The model under review builds one solid part; all positions refer to its coordinate system, in mm. A direction names the side the tool comes from. Coordinates: 2 decimals unless noted, no trailing zeros. Order: outer loops, then holes, each group sorted by start corner. A loop starts at its lowest first (then second) coordinate and runs counter-clockwise, first axis right, second up. Notation, with made-up numbers: M 31.5,0.5 L 89.5,0.5 A16 ccw 89.5,21.5 Z; hole C 70,11.25 d6. An arc over 180 degrees is marked long. One line per item, written item: value.
```python
from build123d import *

# Parameters (mm, degrees)
SKETCH1_W                   = 126
SKETCH1_H                   = 5
ENCAIXE_START               = -7
ENCAIXE_POTENCI_METRO_DEPTH = 7


with BuildPart() as part:
    # Sketch1 → Blank (revolve)
    with BuildSketch(Plane.XY, mode=Mode.PRIVATE) as blank_sk:
        with Locations((0, 2.5)):
            Rectangle(SKETCH1_W, SKETCH1_H)
    revolve(blank_sk.sketch.rotate(Axis((-63, 0, 0), (1, 0, 0)), 90), axis=Axis((-63, 0, 0), (1, 0, 0)))

    # Sketch2 → Encaixe - Potenciômetro (cut)
    with BuildSketch(Plane.ZY.offset(63).offset(ENCAIXE_START)):
        with BuildLine():
            Line((0.25, 4.993746089), (0.25, -4.993746089))
            ThreePointArc((0.25, -4.993746089), (3.622844187, -3.446012188), (5, 0))
            ThreePointArc((5, 0), (3.622844187, 3.446012188), (0.25, 4.993746089))
        make_face()
        with BuildLine():
            ThreePointArc((-0.25, 4.993746089), (-5, 0), (-0.25, -4.993746089))
            Line((-0.25, -4.993746089), (-0.25, 4.993746089))
        make_face()
    extrude(amount=ENCAIXE_POTENCI_METRO_DEPTH, mode=Mode.SUBTRACT)


solid = part.part
```
(1) We need section B-B, the plane x = -4.5. State the section outline as (y, z) points, plus the area to 3 significant figures.
Geometry results:
outline: C 0,0 d10
area: 78.5 mm2
(2) Tool access review of faces 4 (the cylindrical face through (0.882, 1.915, 4.619)), 5 (the flat face through (-59, 0, -0.25)): name each direction out of +Z, -Z, +X, -X, +Y, -Y from which nothing blocks a thin tool from reaching the whole face with its end or side.
Geometry results:
face 4: +X, -X
face 5: -Z, -X, +Y, -Y
(3) We need section D-D, the plane z = -2.75. State the section outline as (x, y) points.
Geometry results:
outline: M -56,-4.18 L 63,-4.18 L 63,4.18 L -56,4.18 Z
(4) Mouldability with a two-part tool opening along X and no side actions: class faces 1 (the flat face through (63, 0, 0)), 2 (the flat face through (-59, 0, 0.25)), 3 (the flat face through (-56, 0, 2)) as +X half, -X half, draft (parallel to the pull), parting line (faces both ways), or undercut.
Geometry results:
face 1: +X half
face 2: draft
face 3: -X half
(5) Insertion check: pin 1 Ø1.5 at (x, z) = (2.5, 3.5) entering from -Y; pin 2 Ø1.5 at (x, y) = (-47.5, 1) entering from +Z; pin 3 Ø1.5 at (x, y) = (-39.5, -1) entering from -Z. Each pin has a flat end and moves straight along its axis. Give the tip position at first contact, or say it passes through.
Geometry results:
pin 1: stops at y = -4.18
pin 2: stops at z = 4.99
pin 3: stops at z = -4.99
(6) For L1, parallel to X at y = -1.5, z = -2.75; L2, parallel to Y at x = 12.5, z = -0.5; L3, parallel to Y at x = -49, z = -2, list the stretches that pass through material, from the lowest coordinate up.
Geometry results:
L1: x = -56 to 63
L2: y = -4.97 to 4.97
L3: y = -4.58 to 4.58
(7) We need section C-C, the plane z = 2.5. State the section outline as (x, y) points.
Geometry results:
outline: M -56,-4.33 L 63,-4.33 L 63,4.33 L -56,4.33 Z
(8) We need section A-A, the plane y = 0. State the section outline as (x, z) points, plus the area to 3 significant figures.
Geometry results:
outline: M -63,-0.25 L -56,-0.25 L -56,-5 L 63,-5 L 63,5 L -56,5 L -56,0.25 L -63,0.25 Z
area: 1,190 mm2
